from build123d import *

# Parameters (mm, degrees)
SKETCH1_R           = 13
SKETCH1_R_2         = 2.75
BOSS_EXTRUDE1_DEPTH = 5
SKETCH2_W           = 11
SKETCH2_H           = 600
BOSS_EXTRUDE2_DEPTH = 3
FILLET1_R           = 20


with BuildPart() as part:
    # Sketch1 → Boss-Extrude1 (new body)
    with BuildSketch(Plane(origin=(0, 0, 0), x_dir=(1, 0, 0), z_dir=(0, 1, 0))):
        Polygon((40, -40), (-40, -40), (-40, 40), (-40, 40.5), (40, 40.5), (40, 40), align=None)
        with Locations(Location((0, 0, 0), (0, 0, 270))):
            Circle(SKETCH1_R, mode=Mode.SUBTRACT)
        with Locations(Location((-17.5, -17.5, 0), (0, 0, 270))):
            Circle(SKETCH1_R_2, mode=Mode.SUBTRACT)
        with Locations(Location((17.5, -17.5, 0), (0, 0, 270))):
            Circle(SKETCH1_R_2, mode=Mode.SUBTRACT)
        with Locations(Location((17.5, 17.5, 0), (0, 0, 270))):
            Circle(SKETCH1_R_2, mode=Mode.SUBTRACT)
        with Locations(Location((-17.5, 17.5, 0), (0, 0, 270))):
            Circle(SKETCH1_R_2, mode=Mode.SUBTRACT)
    extrude(amount=BOSS_EXTRUDE1_DEPTH)

    # Sketch2 → Boss-Extrude2 (add)
    with BuildSketch(Plane(origin=(0, 0, -40.5), x_dir=(-1, 0, 0), z_dir=(0, 0, -1))):
        with Locations((9.5, -295)):
            Rectangle(SKETCH2_W, SKETCH2_H)
        with Locations((-9.5, -295)):
            Rectangle(SKETCH2_W, SKETCH2_H)
    extrude(amount=-BOSS_EXTRUDE2_DEPTH)

    # Fillet1
    fillet1_edges = [part.edges().sort_by_distance(p)[0] for p in [
        (40, 2.5, 40),
        (-40, 2.5, 40),
    ]]
    fillet(fillet1_edges, radius=FILLET1_R)


solid = part.part
Read the model definition and answer for the solid it produces. Units are mm, in the model's axes. A direction names the side the tool comes from. Round coordinates to 2 decimals unless told otherwise and drop trailing zeros. Loops run counter-clockwise (first coordinate to the right, second up) from the corner with the lowest first, then second, coordinate; pieces in that order, holes last. Notation, with made-up numbers: (28, -39) - (86, -39) arc R31 cw to (86, -15) - close; hole circle Ø10 at (-16, 40). An arc over 180 degrees is marked (long way). One line per question, with ' | ' between items. Start each with the question number.
Q1. For a pull along X with two mould halves and no side action, classify faces 3 (the cylindrical face through (33.986, 2.535, 34.297)), 4 (the cylindrical face through (-7.91, 2.465, -10.316)), 5 (the flat face through (9, 5, -10)) as +X half, -X half, draft (parallel to the pull), parting line (faces both ways), or undercut.
Q2. For faces 1 (the cylindrical face through (-33.986, 2.535, 34.297)), 2 (the flat face through (-9, -293, -37.5)), determine the directions among +Z, -Z, +X, -X, +Y, -Y from which every point of the face is accessible in a straight line to the end or side of a thin tool.
Q3. Find the intervals of material crossed by L1, parallel to X at y = 1.5, z = 17.5; L2, parallel to Z at x = -17, y = 2; L3, parallel to X at y = 1, z = 0, in increasing order.
Q4. Section A-A on z = 5 is taken. Give the vertices of the cut face in (x, y).
Q5. Flat-ended cylindrical pins translate along their axes: pin 1 (1.5 mm diameter, centred on x = 31.5, z = 24.5, fed in from -Y); pin 2 (4.5 mm diameter, centred on x = 17.5, z = -17.5, fed in from +Y); pin 3 (2.5 mm diameter, centred on y = -328.5, z = -39, fed in from +X); pin 4 (1.5 mm diameter, centred on y = -442, z = -39, fed in from -X). Find the tip coordinate at first contact, or state that the pin passes through.
Q6. Section C-C on x = 34 is taken. Give the vertices of the cut face in (y, z).
Q7. Section B-B on y = -460.5 is taken. Give the vertices of the cut face in (x, z), plus the area to 3 significant figures.
Established:
1) face 3: +X half | face 4: undercut | face 5: draft
2) face 1: +Z, -X, +Y, -Y | face 2: +Z, +X, -X, -Y
3) L1: -40 to -20.25, -14.75 to 14.75, 20.25 to 40 | L2: -40.5 to -20.2, -14.8 to 14.8, 20.2 to 40 | L3: -40 to -13, 13 to 40
4) outline: (-40, 0) - (-12, 0) - (-12, 5) - (-40, 5) - close; (12, 0) - (40, 0) - (40, 5) - (12, 5) - close
5) pin 1: y = 0 | pin 2: through | pin 3: x = 15 | pin 4: x = -15
6) outline: (0, -40.5) - (5, -40.5) - (5, 34.28) - (0, 34.28) - close
7) outline: (-15, -40.5) - (-4, -40.5) - (-4, -37.5) - (-15, -37.5) - close; (4, -40.5) - (15, -40.5) - (15, -37.5) - (4, -37.5) - close | area: 66.0 mm²
